Solid Edge part; units mm, degrees
sketch "Sketch1" plane through (0, 0, 0) normal (0, -1, 0) x (1, 0, 0)
  line L0 (19.05, 22.25) -> (-19.05, 22.25)
  line L1 (-19.05, 22.25) -> (-19.05, -22.25)
  line L2 (-19.05, -22.25) -> (19.05, -22.25)
  line L3 (19.05, -22.25) -> (19.05, 22.25)
extrude "Protrusion1" add sketch "Sketch1" against normal blind 38.1
sketch "Sketch2" plane through (19.05, 19.05, 0) normal (1, 0, 0) x (0, 1, 0)
  line L0 (12.0974, 22.25) -> (19.05, 22.25)
  line L1 (19.05, 22.25) -> (19.05, -9.55)
  arc A0 (19.05, -9.55) -> (12.0974, 22.25) centre (-57.15, -9.55) ccw
extrude "ExtrudedCutout_2" cut sketch "Sketch2" against normal blind 42
CAD build for the part. Positions are in the model's coordinates, mm. Give positions to 0.01 mm unless a question says otherwise; leave off trailing zeros. Order: outer loops, then holes, each group sorted by start corner. A loop starts at its lowest first (then second) coordinate and runs counter-clockwise, first axis right, second up. Notation, with made-up numbers: M 10,-18.75 L 50,-18.75 A14 ccw 50,4.25 Z; hole C 22.5,14 d6. An arc over 180 degrees is marked long. Put each result on its own line as item: value. Start each with the question number.
(1) Saw through at B-B, the plane z = 8.5. Write the cut outline in (x, y).
(2) Drill centre lines: line 1 along Y through (x, z) = (11.5, 8); line 2 along Y through (x, z) = (15.5, 11.5); line 3 along Z through (x, y) = (16.5, 32). Where is each one in solid material? Low to high.
(3) Saw through at A-A, the plane x = 1.5. Write the cut outline in (y, z).
(4) Flat gauge pin, fed straight in: pin 1 Ø1 at (x, z) = (10, -6) entering from +Y. Where does the tip first touch, or does it go through?
(5) Saw through at C-C, the plane z = 19.5. Write the cut outline in (x, y), then the cut area to 3 significant figures.
Check result:
1. outline: M -19.05,0 L 19.05,0 L 19.05,35.93 L -19.05,35.93 Z
2. line 1: y = 0 to 36.05
2. line 2: y = 0 to 35.13
2. line 3: z = -22.25 to 20.32
3. outline: M 0,-22.25 L 38.1,-22.25 L 38.1,-9.55 A76.2 ccw 31.15,22.25 L 0,22.25 Z
4. pin 1: stops at y = 38.04
5. outline: M -19.05,0 L 19.05,0 L 19.05,32.35 L -19.05,32.35 Z
5. area: 1,230 mm2
